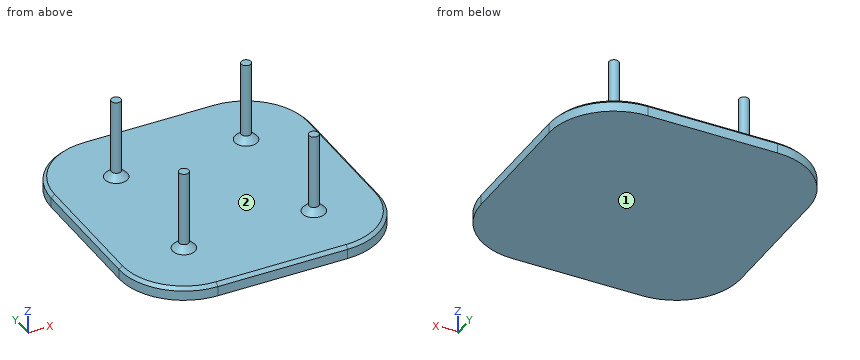
```python
from build123d import *

# Parameters (mm, degrees)
SKETCH_W        = 80
SKETCH_H        = 80
PAD_DEPTH       = 4
SKETCH001_R     = 1.5
PAD001_DEPTH    = 25
FILLET_R        = 20
CHAMFER_SIZE    = 2
CHAMFER001_SIZE = 1


with BuildPart() as part:
    # Sketch → Pad (new body)
    with BuildSketch(Plane.XY):
        with Locations((40, 40)):
            Rectangle(SKETCH_W, SKETCH_H)
    extrude(amount=PAD_DEPTH)

    # Sketch001 (on Face6 of Pad) → Pad001 (join)
    with BuildSketch(Plane.XY.offset(4)):
        with Locations((20, 60)):
            Circle(SKETCH001_R)
        with Locations((60, 60)):
            Circle(SKETCH001_R)
        with Locations((20, 20)):
            Circle(SKETCH001_R)
        with Locations((60, 20)):
            Circle(SKETCH001_R)
    extrude(amount=PAD001_DEPTH)

    # Fillet
    fillet_edges = [part.edges().sort_by_distance(p)[0] for p in [
        (80, 0, 2),
        (80, 80, 2),
        (0, 0, 2),
        (0, 80, 2),
    ]]
    fillet(fillet_edges, radius=FILLET_R)

    # Chamfer
    chamfer_edges = [part.edges().sort_by_distance(p)[0] for p in [
        (18.5, 60, 4),
        (18.5, 20, 4),
        (58.5, 20, 4),
        (58.5, 60, 4),
    ]]
    chamfer(chamfer_edges, length=CHAMFER_SIZE)

    # Chamfer001
    chamfer001_edges = [part.edges().sort_by_distance(p)[0] for p in [
        (0, 40, 4),
        (5.857864, 5.857864, 4),
        (40, 0, 4),
        (74.142136, 5.857864, 4),
        (80, 40, 4),
        (74.142136, 74.142136, 4),
        (40, 80, 4),
        (5.857864, 74.142136, 4),
    ]]
    chamfer(chamfer001_edges, length=CHAMFER001_SIZE)


solid = part.part
```
Source: CAD feature listing. Evaluate the final solid. Frame: model axes, mm. Face numbers are marked on the shaded views. A direction names the side the tool comes from. Round coordinates to 2 decimals unless told otherwise and drop trailing zeros. Loops run counter-clockwise (first coordinate to the right, second up) from the corner with the lowest first, then second, coordinate; pieces in that order, holes last.
1. Contact query for flat-ended pins moving along their axis: pin 1 (4 mm diameter, centred on x = 63, z = 12.5, fed in from +Y); pin 2 (12 mm diameter, centred on x = 66, z = 14.5, fed in from +Y); pin 3 (6 mm diameter, centred on y = 23.5, z = 22.5, fed in from +X). Output: stop coordinate, or through.
2. Ray query, L1, parallel to Z at x = 21.5, y = 26; L2, parallel to X at y = 61, z = 23; L3, parallel to Y at x = 66, z = 3.5. Return the intervals inside material, ascending.
3. Section query B-B on x = 44. Output: boundary loops of the cut face in (y, z), and give its area (3 significant figures).
4. Access query for the marked faces 1 and 2. Directions: +Z, -Z, +X, -X, +Y, -Y. A direction counts if a zero-diameter tool reaches every point of the face in a straight line with its end or side. Return the directions, or none.
5. Section query A-A on z = 14. Output: boundary loops of the cut face in (x, y).
Answers below:
1. pin 1: stops at y = 61.12
1. pin 2: stops at y = 61.5
1. pin 3: stops at x = 61.41
2. L1: z = 0 to 4
2. L2: x = 18.88 to 21.12, 58.88 to 61.12
2. L3: y = 1.45 to 78.55
3. outline: (0, 0) - (80, 0) - (80, 3) - (79, 4) - (1, 4) - (0, 3) - close
3. area: 319 mm2
4. face 1: -Z, +X, -X, +Y, -Y
4. face 2: +Z
5. outline: circle Ø3 at (20, 20); circle Ø3 at (20, 60); circle Ø3 at (60, 20); circle Ø3 at (60, 60)
